For this review, take the finished solid that the model builds, in its own axes (mm). Face numbers are marked on the shaded views. A direction names the side the tool comes from. Round coordinates to 2 decimals unless told otherwise and drop trailing zeros. Order: outer loops, then holes, each group sorted by start corner. A loop starts at its lowest first (then second) coordinate and runs counter-clockwise, first axis right, second up. Notation, with made-up numbers: M -1.75,45.25 L 4.25,45.25 A20 ccw 4.25,57.25 Z; hole C -28,-5 d2. An arc over 180 degrees is marked long. Answer as a JSON object with one key per item and string values.
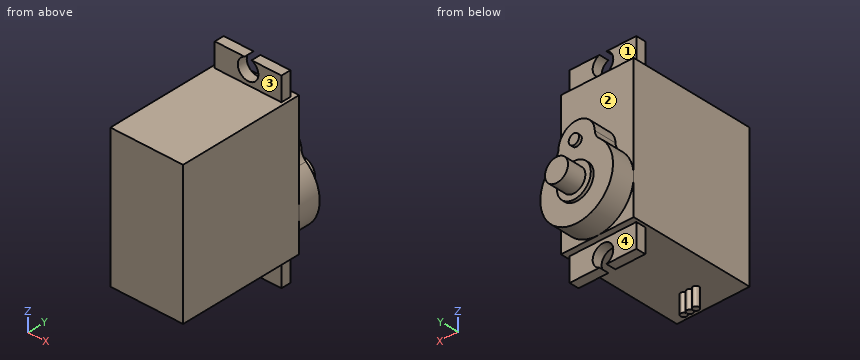
from build123d import *

# Parameters (mm, degrees)
SKETCH1_W                = 12
SKETCH1_H                = 23.2
BOSS_EXTRUDE1_DEPTH      = 20.7
SKETCH2_W                = 11
SKETCH2_H                = 1.6
BOSS_EXTRUDE2_DEPTH      = 3.9
SKETCH3_W                = 11
SKETCH3_H                = 1.6
BOSS_EXTRUDE3_DEPTH      = 3.9
SKETCH4_R                = 6
BOSS_EXTRUDE4_DEPTH      = 3.7
SKETCH5_R                = 3
BOSS_EXTRUDE5_DEPTH      = 3.7
FILLET1_R                = 2
SKETCH6_R                = 0.85
BOSS_EXTRUDE6_DEPTH      = 0.5
SKETCH7_R                = 2.8
BOSS_EXTRUDE7_DEPTH      = 0.5
SKETCH8_R                = 1.9
BOSS_EXTRUDE8_DEPTH      = 3.1
M3_CLEARANCE_HOLE1_D     = 3.4
M3_CLEARANCE_HOLE1_DEPTH = 3
M3_CLEARANCE_HOLE1_TIP   = 1.021463052
SKETCH11_R               = 0.5
BOSS_EXTRUDE9_DEPTH      = 3
LPATTERN2_COUNT          = 3
LPATTERN2_PITCH          = 1.01


with BuildPart() as part:
    # Sketch1 → Boss-Extrude1 (new body)
    with BuildSketch(Plane(origin=(0, 0, 0), x_dir=(1, 0, 0), z_dir=(0, 1, 0))):
        with Locations((6, 11.6)):
            Rectangle(SKETCH1_W, SKETCH1_H)
    extrude(amount=BOSS_EXTRUDE1_DEPTH)

    # Sketch2 → Boss-Extrude2 (add)
    with BuildSketch(Plane.XY):
        with Locations((6, 18.9)):
            Rectangle(SKETCH2_W, SKETCH2_H)
    extrude(amount=BOSS_EXTRUDE2_DEPTH)

    # Sketch3 → Boss-Extrude3 (add)
    with BuildSketch(Plane(origin=(0, 0, -23.2), x_dir=(-1, 0, 0), z_dir=(0, 0, -1))):
        with Locations((-6, 18.9)):
            Rectangle(SKETCH3_W, SKETCH3_H)
    extrude(amount=BOSS_EXTRUDE3_DEPTH)

    # Sketch4 → Boss-Extrude4 (add)
    with BuildSketch(Plane(origin=(0, 20.7, 0), x_dir=(1, 0, 0), z_dir=(0, 1, 0))):
        with Locations(Location((6, 17.2, 0), (0, 0, 90))):
            Circle(SKETCH4_R)
    extrude(amount=BOSS_EXTRUDE4_DEPTH)

    # Sketch5 → Boss-Extrude5 (add)
    with BuildSketch(Plane(origin=(0, 20.7, 0), x_dir=(1, 0, 0), z_dir=(0, 1, 0))):
        with Locations((6, 11.2)):
            Circle(SKETCH5_R)
    extrude(amount=BOSS_EXTRUDE5_DEPTH)

    # Fillet1
    fillet1_edges = [part.edges().sort_by_distance(p)[0] for p in [
        (3.09526249, 22.55, -11.95),
        (8.90473751, 22.55, -11.95),
    ]]
    fillet(fillet1_edges, radius=FILLET1_R)

    # Sketch6 → Boss-Extrude6 (add)
    with BuildSketch(Plane(origin=(0, 24.4, 0), x_dir=(1, 0, 0), z_dir=(0, 1, 0))):
        with Locations(Location((6, 11.2, 0), (0, 0, 270))):
            Circle(SKETCH6_R)
    extrude(amount=BOSS_EXTRUDE6_DEPTH)

    # Sketch7 → Boss-Extrude7 (add)
    with BuildSketch(Plane(origin=(0, 24.4, 0), x_dir=(1, 0, 0), z_dir=(0, 1, 0))):
        with Locations(Location((6, 17.2, 0), (0, 0, 270))):
            Circle(SKETCH7_R)
    extrude(amount=BOSS_EXTRUDE7_DEPTH)

    # Sketch8 → Boss-Extrude8 (add)
    with BuildSketch(Plane(origin=(0, 24.9, 0), x_dir=(1, 0, 0), z_dir=(0, 1, 0))):
        with Locations(Location((6, 17.2, 0), (0, 0, 90))):
            Circle(SKETCH8_R)
    extrude(amount=BOSS_EXTRUDE8_DEPTH)

    # M3 Clearance Hole1
    with Locations(Plane(origin=(0, 19.7, 0), x_dir=(1, 0, 0), z_dir=(0, 1, 0))):
        with Locations((6, -2.3), (6, 25.5)):
            Hole(M3_CLEARANCE_HOLE1_D / 2, depth=M3_CLEARANCE_HOLE1_DEPTH)
            with Locations((0, 0, -(M3_CLEARANCE_HOLE1_DEPTH + M3_CLEARANCE_HOLE1_TIP / 2))):  # 118° drill point
                Cone(0, M3_CLEARANCE_HOLE1_D / 2, M3_CLEARANCE_HOLE1_TIP, mode=Mode.SUBTRACT)

    # Sketch11 → Boss-Extrude9 (add)
    with BuildSketch(Plane(origin=(0, 0, -23.2), x_dir=(-1, 0, 0), z_dir=(0, 0, -1))):
        with Locations(Location((-7, 4.2, 0), (0, 0, 180))):
            Circle(SKETCH11_R)
    boss_extrude9 = extrude(amount=BOSS_EXTRUDE9_DEPTH)

    # LPattern2: Boss-Extrude9 ×3
    with Locations(*[(-i * LPATTERN2_PITCH, 0, 0) for i in range(1, LPATTERN2_COUNT)]):
        add(boss_extrude9)


solid = part.part
1) For L1, parallel to X at y = 19.2, z = 2.3; L2, parallel to Z at x = 5, y = 18.5; L3, parallel to Y at x = 9.5, z = -22, list the stretches that pass through material, from the lowest coordinate up.
Geometry check:
{"L1": "x = 0.5 to 4.3, 7.7 to 11.5", "L2": "z = -27.1 to -26.87, -24.13 to 0.93, 3.67 to 3.9", "L3": "y = 0 to 24.4"}
2) Machinability: for the marked faces 1, 2, 3 and 4, which of the approach directions +Z, -Z, +X, -X, +Y, -Y give a long, thin tool a straight path to every point of the face, cutting with its end or side? Answer none if there is none.
Geometry check:
{"face 1": "+Z, +X, -X, +Y", "face 2": "+Z, +Y", "face 3": "+Z, +X, -X, -Y", "face 4": "-Z, +X, -X, +Y"}
3) Add section B-B on z = 1.5. State the section outline as (x, y) points.
Geometry check:
{"outline": "M 0.5,18.1 L 4.5,18.1 L 4.5,19.7 L 0.5,19.7 Z; M 7.5,18.1 L 11.5,18.1 L 11.5,19.7 L 7.5,19.7 Z"}
4) Insertion check: P1, Ø0.5, axis at x = 5, y = 4, coming from the -Z side; P2, Ø1.5, axis at x = 2, y = 13.5, coming from the -Z side; P3, Ø6.5, axis at x = 2, z = -19, coming from the +Y side; P4, Ø3, axis at x = 6, z = -25.5, coming from the -Y side. Each pin has a flat end and moves straight along its axis. Give the tip position at first contact, or say it passes through.
Geometry check:
{"P1": "stops at z = -26.2", "P2": "stops at z = -23.2", "P3": "stops at y = 28", "P4": "stops at y = 3.7"}
5) Add section D-D on z = -2. State the section outline as (x, y) points, and give its area (3 significant figures).
Geometry check:
{"outline": "M 0,0 L 12,0 L 12,20.7 L 0,20.7 Z", "area": "248 mm²"}
6) Add section A-A on z = -25.5. State the section outline as (x, y) points, and give its area (3 significant figures).
Geometry check:
{"outline": "M 0.5,18.1 L 4.3,18.1 L 4.3,19.7 L 0.5,19.7 Z; C 4.98,4.2 d1; C 5.99,4.2 d1; C 7,4.2 d1; M 7.7,18.1 L 11.5,18.1 L 11.5,19.7 L 7.7,19.7 Z", "area": "14.5 mm²"}
